```python
from build123d import *

# Parameters (mm, degrees)
SKETCH2_R                                      = 30.2
BOSS_EXTRUDE1_DEPTH                            = 425
SKETCH3_R                                      = 26.2
CUT_EXTRUDE1_DEPTH                             = 426
CUT_EXTRUDE2_REACH                             = 32.2
SKETCH4_W                                      = 60.4
SKETCH4_H                                      = 425
CSK_FOR_M6_FLAT_HEAD_MACHINE_SCREW1_AT_2_COUNT = 2
CSK_FOR_M6_FLAT_HEAD_MACHINE_SCREW1_AT_2_PITCH = 90
CSK_FOR_M6_FLAT_HEAD_MACHINE_SCREW1_AT_3_COUNT = 2
CSK_FOR_M6_FLAT_HEAD_MACHINE_SCREW1_AT_3_PITCH = 180
CSK_FOR_M6_FLAT_HEAD_MACHINE_SCREW1_AT_4_COUNT = 2
CSK_FOR_M6_FLAT_HEAD_MACHINE_SCREW1_AT_4_PITCH = 270
CSK_FOR_M6_FLAT_HEAD_MACHINE_SCREW1_AT_5_COUNT = 2
CSK_FOR_M6_FLAT_HEAD_MACHINE_SCREW1_AT_5_PITCH = 360


with BuildPart() as part:
    # Sketch2 → Boss-Extrude1 (new body)
    with BuildSketch(Plane.XY):
        Circle(SKETCH2_R)
    extrude(amount=-BOSS_EXTRUDE1_DEPTH)

    # Sketch3 → Cut-Extrude1 (cut, through all)
    with BuildSketch(Plane.XY):
        Circle(SKETCH3_R)
    extrude(amount=-CUT_EXTRUDE1_DEPTH, mode=Mode.SUBTRACT)

    # Sketch4 → Cut-Extrude2 (cut, up to next)
    with BuildSketch(Plane(origin=(0, 0, 0), x_dir=(1, 0, 0), z_dir=(0, 1, 0)), mode=Mode.PRIVATE) as cut_extrude2_sk1:
        with Locations((0, 212.5)):
            Rectangle(SKETCH4_W, SKETCH4_H)
    cut_extrude2_tool1 = extrude(cut_extrude2_sk1.sketch, amount=-CUT_EXTRUDE2_REACH, mode=Mode.PRIVATE) & part.part
    add(cut_extrude2_tool1.solids().sort_by_distance((0, 0, -212.5))[0], mode=Mode.SUBTRACT)

    # Sketch10 → CSK for M6 Flat Head Machine Screw1 (revolve, cut)
    with BuildSketch(Plane(origin=(0, 0, -40), x_dir=(0, 0, -1), z_dir=(1, 0, 0))):
        Polygon((0, 0), (0, 30.2), (3.5, 30.2), (3.5, 28.8), (6.3, 26), (6.3, 0), align=None)
    csk_for_m6_flat_head_machine_screw1 = revolve(axis=Axis((0, -6.35, -40), (0, 1, 0)), mode=Mode.SUBTRACT)

    # CSK for M6 Flat Head Machine Screw1 at 2: CSK for M6 Flat Head Machine Screw1 ×2
    with Locations(*[(0, 0, -i * CSK_FOR_M6_FLAT_HEAD_MACHINE_SCREW1_AT_2_PITCH) for i in range(1, CSK_FOR_M6_FLAT_HEAD_MACHINE_SCREW1_AT_2_COUNT)]):
        add(csk_for_m6_flat_head_machine_screw1, mode=Mode.SUBTRACT)

    # CSK for M6 Flat Head Machine Screw1 at 3: CSK for M6 Flat Head Machine Screw1 ×2
    with Locations(*[(0, 0, -i * CSK_FOR_M6_FLAT_HEAD_MACHINE_SCREW1_AT_3_PITCH) for i in range(1, CSK_FOR_M6_FLAT_HEAD_MACHINE_SCREW1_AT_3_COUNT)]):
        add(csk_for_m6_flat_head_machine_screw1, mode=Mode.SUBTRACT)

    # CSK for M6 Flat Head Machine Screw1 at 4: CSK for M6 Flat Head Machine Screw1 ×2
    with Locations(*[(0, 0, -i * CSK_FOR_M6_FLAT_HEAD_MACHINE_SCREW1_AT_4_PITCH) for i in range(1, CSK_FOR_M6_FLAT_HEAD_MACHINE_SCREW1_AT_4_COUNT)]):
        add(csk_for_m6_flat_head_machine_screw1, mode=Mode.SUBTRACT)

    # CSK for M6 Flat Head Machine Screw1 at 5: CSK for M6 Flat Head Machine Screw1 ×2
    with Locations(*[(0, 0, -i * CSK_FOR_M6_FLAT_HEAD_MACHINE_SCREW1_AT_5_PITCH) for i in range(1, CSK_FOR_M6_FLAT_HEAD_MACHINE_SCREW1_AT_5_COUNT)]):
        add(csk_for_m6_flat_head_machine_screw1, mode=Mode.SUBTRACT)


solid = part.part
```
Part model, mm, in its own coordinate system. Coordinates: 2 decimals unless noted, no trailing zeros. Loops run counter-clockwise (first coordinate to the right, second up) from the corner with the lowest first, then second, coordinate; pieces in that order, holes last. Notation, with made-up numbers: (-26.5, 14) - (29.5, 14) arc R20 cw to (29.5, 31) - close; hole circle Ø1 at (45.5, 50). An arc over 180 degrees is marked (long way). Write item = value, one per line. Start each with the question number.
Item 1: Cut at A-A, the plane y = 15.5. Give the cut face in (x, z), and give its area (3 significant figures).
Item 2: Cut at D-D, the plane z = -199.5. Give the cut face in (x, y), and give its area (3 significant figures).
Item 3: Flat gauge pins, fed straight in: pin 1 Ø1 at (x, z) = (-19, -254) entering from -Y; pin 2 Ø5 at (x, z) = (-15, -136.5) entering from -Y; pin 3 Ø11 at (x, z) = (0, -130) entering from -Y; pin 4 Ø12 at (x, y) = (17, 15.5) entering from -Z. Where does each tip first touch, or does it go through?
Item 4: Cut at B-B, the plane z = -400. Give the cut face in (x, y).
Item 5: Cut at C-C, the plane x = -14.5. Give the cut face in (y, z), and give its area (3 significant figures).
Item 6: Wall check: L1, parallel to Z at x = 0, y = 29.2; L2, parallel to X at y = 10.5, z = -59; L3, parallel to Y at x = 0.5, z = -46.5. Give the ranges that are in metal, low to high. Write a range as from..to.
Item 7: Mould opens along Z. For faces 1 (the conical face through (-1.1, 28.62, -43.51)), 2 (the flat face through (-0.1, 26.4, 0)), 3 (the cylindrical face through (3.105, 29.49, -131.615)), 4 (the flat face through (-0.1, 26.4, -425)) say: released by +Z, released by -Z, zero draft, split by the parting line, or undercut.
The answers:
q1.outline = (-25.92, -425) - (-21.12, -425) - (-21.12, 0) - (-25.92, 0) - close; (21.12, -425) - (25.92, -425) - (25.92, 0) - (21.12, 0) - close
q1.area = 4,080 mm2
q2.outline = (-30.2, 0) - (-26.2, 0) arc R26.2 cw to (26.2, 0) - (30.2, 0) arc R30.2 ccw to start
q2.area = 354 mm2
q3.pin_1 = 17.5
q3.pin_2 = 19.5
q3.pin_3 = 26.8
q3.pin_4 = -425
q4.outline = (-30.2, 0) - (-26.2, 0) arc R26.2 cw to (-6.3, 25.43) - (-6.3, 26) - (-3.5, 28.8) - (-3.5, 30) arc R30.2 ccw to start; (3.5, 28.8) - (6.3, 26) - (6.3, 25.43) arc R26.2 cw to (26.2, 0) - (30.2, 0) arc R30.2 ccw to (3.5, 30) - close
q5.outline = (21.82, -425) - (26.49, -425) - (26.49, 0) - (21.82, 0) - close
q5.area = 1,980 mm2
q6.L1 = -425..-403.5, -396.5..-313.5, -306.5..-223.5, -216.5..-133.5, -126.5..-43.5, -36.5..0
q6.L2 = -28.32..-24, 24..28.32
q6.L3 = 26.2..30.2
q7.face_1 = undercut
q7.face_2 = released by +Z
q7.face_3 = undercut
q7.face_4 = released by -Z
